```python
from build123d import *

# Parameters (mm, degrees)
FILLET1_R          = 1
SKETCH2_R          = 2.5
SKETCH2_R_2        = 1
CUT_EXTRUDE1_DEPTH = 5


with BuildPart() as part:
    # Sketch1 → Revolve1 (revolve)
    with BuildSketch(Plane(origin=(0, 0, 0), x_dir=(1, 0, 0), z_dir=(0, 1, 0))):
        with BuildLine():
            Line((5.429394359, 13), (4.429394359, 13))
            Line((4.429394359, 13), (4.429394359, 11.9))
            Line((4.429394359, 11.9), (-3.070605641, 11.9))
            Line((-3.070605641, 11.9), (-3.070605641, 9.9))
            Line((-3.070605641, 9.9), (0.164577559, 9.9))
            Line((0.164577559, 9.9), (0.164577559, 7.086841674))
            Line((0.164577559, 7.086841674), (0.164577559, 3.25))
            Line((0.164577559, 3.25), (-4.835422441, 3.25))
            Line((-4.835422441, 3.25), (-4.835422441, 1.25))
            Line((-4.835422441, 1.25), (1.847087525, 1.25))
            Line((1.847087525, 1.25), (1.847087525, 0))
            Line((1.847087525, 0), (3.847087525, 0))
            Line((3.847087525, 0), (3.847087525, 7.12829034))
            ThreePointArc((3.847087525, 7.12829034), (3.753395312, 7.550908601), (3.489875135, 7.894334783))
            Line((3.489875135, 7.894334783), (2.164577559, 9.086841674))
            Line((2.164577559, 9.086841674), (1.664577559, 9.086841674))
            Line((1.664577559, 9.086841674), (1.664577559, 9.586841674))
            Line((1.664577559, 9.586841674), (2.164577559, 9.586841674))
            Line((2.164577559, 9.586841674), (2.164577559, 11.086841674))
            Line((2.164577559, 11.086841674), (5.164577559, 11.086841674))
            Line((5.164577559, 11.086841674), (5.164577559, 12.5))
            Line((5.164577559, 12.5), (5.429394359, 12.5))
            Line((5.429394359, 12.5), (5.429394359, 13))
        make_face()
    revolve(axis=Axis((-7.139696802, 0, 0), (1, 0, 0)))

    # Fillet1
    fillet1_edges = [part.edges().sort_by_distance(p)[0] for p in [
        (5.164577559, 0, 11.086841674),
    ]]
    fillet(fillet1_edges, radius=FILLET1_R)

    # Sketch2 → Cut-Extrude1 (cut, symmetric)
    with BuildSketch(Plane(origin=(3.847087525, 0, 0), x_dir=(0, 0, -1), z_dir=(1, 0, 0))):
        Circle(SKETCH2_R)
        with Locations((0, 4.68715006)):
            Circle(SKETCH2_R_2)
        with Locations((4.68715006, 0)):
            Circle(SKETCH2_R_2)
        with Locations((0, -4.68715006)):
            Circle(SKETCH2_R_2)
        with Locations((-4.68715006, 0)):
            Circle(SKETCH2_R_2)
    extrude(amount=CUT_EXTRUDE1_DEPTH, both=True, mode=Mode.SUBTRACT)


solid = part.part
```
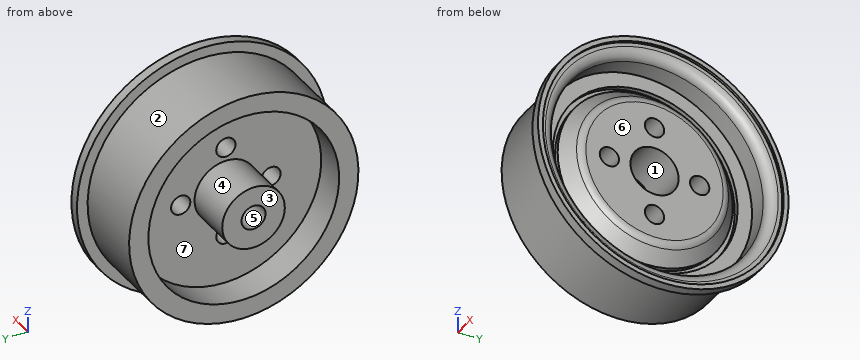
Part model, mm, in its own coordinate system. Face numbers are marked on the shaded views. A direction names the side the tool comes from. Round coordinates to 2 decimals unless told otherwise and drop trailing zeros.
Item 1: Cut at A-A, the plane z = 0. State how many separate pieces and enclosed holes the cut face has, then the cut area to 3 significant figures.
Item 2: Drop flat-ended pins along their axis: P1, Ø4, axis at x = -0.5, z = 1, coming from the -Y side; P2, Ø2, axis at y = 4.5, z = -8.5, coming from the +X side; P3, Ø1.8, axis at y = 0, z = 4.69, coming from the -X side; P4, Ø6, axis at y = -8.5, z = -1, coming from the +X side. Give the stop position or say it passes through.
Item 3: 3-axis set-ups, long thin cutter, end or side, ignore diameter. For the marked faces 5, 6 and 7: which of +Z, -Z, +X, -X, +Y, -Y reach the whole face in a straight line?
Item 4: Drill centre lines: line 1 (Y direction, x = 0, z = 0); line 2 (Y direction, x = 1.95, z = 0); line 3 (Y direction, x = 5.3, z = 0). Where is each one in solid material? Low to high.
Item 5: Mould opens along Z. For the marked faces 1, 2, 3 and 4 say: +Z half, -Z half, draft (parallel to the pull), parting line (faces both ways), or undercut.
A:
1. separate pieces: 4
1. enclosed holes: 0
1. area: 77.9 mm2
2. P1: stops at y = -11.9
2. P2: stops at x = 2.69
2. P3: passes through
2. P4: stops at x = 5.01
3. face 5: +X, -X
3. face 6: +X
3. face 7: -X
4. line 1: y = -11.9 to -9.9, -3.25 to -2.5, 2.5 to 3.25, 9.9 to 11.9
4. line 2: y = -11.9 to -9.59, -9.09 to -5.69, -3.69 to -2.5, 2.5 to 3.69, 5.69 to 9.09, 9.59 to 11.9
4. line 3: y = -13 to -12.5, 12.5 to 13
5. face 1: undercut
5. face 2: parting line
5. face 3: draft
5. face 4: undercut
